Source: CAD feature listing. Evaluate the final solid. Frame: model axes, mm. Face numbers are marked on the shaded views. A direction names the side the tool comes from. Give positions to 0.01 mm unless a question says otherwise; leave off trailing zeros. Write each loop counter-clockwise with the first axis right and the second up, starting at its lowest first coordinate (ties: lowest second). Pieces come first, ordered by that corner, then holes. Notation, with made-up numbers: M 36.5,-2 L 74.5,-2 A26 cw 74.5,21 Z; hole C 72.5,67.5 d1. An arc over 180 degrees is marked long. Return JSON: item names as keys, results as strings.
```python
from build123d import *

# Parameters (mm, degrees)
F1_DEPTH = 30
F2_W     = 20
F2_H     = 20
F3_DEPTH = 20
F4_R     = 2
F5_W     = 6
F5_H     = 6
F6_DEPTH = 10
F7_R     = 2.9972
F8_R     = 1.9939
F9_DEPTH = 6


with BuildPart() as f1:
    # F0 (on Top) → F1 (new body)
    with BuildSketch(Plane.XY):
        Polygon((-21.213203, 21.213203), (0, 0), (21.213203, 21.213203), (0, 42.426407), align=None)
    extrude(amount=F1_DEPTH)

    # F2 (on face) → F3 (cut)
    with BuildSketch(Plane(origin=(0, 0, 0), x_dir=(0.707107, -0.707107, 0), z_dir=(-0.707107, -0.707107, 0))):
        with Locations((-15, 15)):
            Rectangle(F2_W, F2_H)
    extrude(amount=-F3_DEPTH, mode=Mode.SUBTRACT)

    # F4
    f4_edges = [f1.edges().sort_by_distance(p)[0] for p in [
        (0, 42.426407, 15),
        (-21.213203, 21.213203, 15),
        (-10.606602, 31.819805, 0),
        (-10.606602, 31.819805, 30),
        (-10.606602, 10.606602, 30),
        (10.606602, 10.606602, 30),
        (10.606602, 31.819805, 30),
        (0, 0, 15),
        (21.213203, 21.213203, 15),
        (10.606602, 10.606602, 0),
        (10.606602, 31.819805, 0),
        (-10.606602, 10.606602, 0),
    ]]
    fillet(f4_edges, radius=F4_R)

    # F5 (on face) → F6 (join)
    with BuildSketch(Plane(origin=(21.213203, 21.213203, 0), x_dir=(-0.707107, 0.707107, 0), z_dir=(0.707107, 0.707107, 0))):
        with Locations((15, 15)):
            Rectangle(F5_W, F5_H)
    extrude(amount=F6_DEPTH)

    # F7
    f7_edges = [f1.edges().sort_by_distance(p)[0] for p in [
        (19.79899, 36.769553, 15),
        (15.556349, 41.012193, 15),
    ]]
    fillet(f7_edges, radius=F7_R)

    # F8 (on face) → F9 (cut)
    with BuildSketch(Plane(origin=(0, 0, 12), x_dir=(1, 0, 0), z_dir=(0, 0, -1))):
        with Locations((15.556349, -36.773512)):
            Circle(F8_R)
    extrude(amount=-F9_DEPTH, mode=Mode.SUBTRACT)


solid = f1.part
```
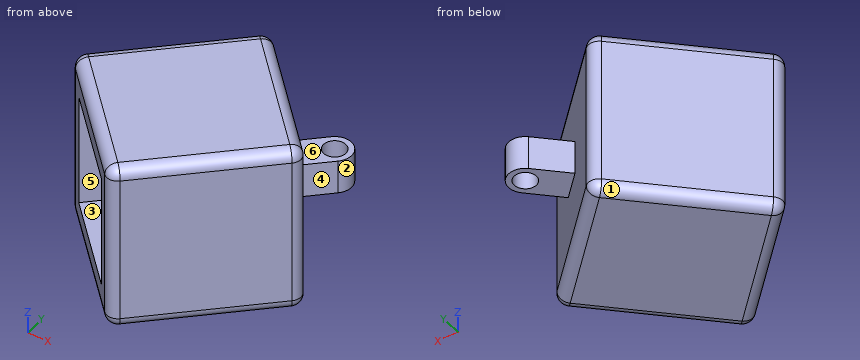
1) Contact query for flat-ended pins moving along their axis: pin 1 Ø6.5 at (x, y) = (15.56, 36.77) entering from -Z; pin 2 Ø6 at (x, z) = (10, 18.5) entering from +Y; pin 3 Ø2 at (x, z) = (-9.5, 25.5) entering from -Y; pin 4 Ø3 at (x, z) = (-1.5, 5.5) entering from -Y. Output: stop coordinate, or through.
Numbers:
{"pin 1": "stops at z = 12", "pin 2": "stops at y = 38.41", "pin 3": "stops at y = 8.5", "pin 4": "stops at y = 0.83"}
2) Set-up query: the marked faces 4, 5 and 6. Return all of +Z, -Z, +X, -X, +Y, -Y with unobstructed straight access to the full face (end or side cutting, diameter ignored); none if empty.
Numbers:
{"face 4": "+Z, -Z, +X", "face 5": "-Y", "face 6": "+Z, +X, +Y"}
3) Draft query along Z for the marked faces 1, 2 and 3. Return one class per face: released by +Z, released by -Z, zero draft, split by the parting line, or undercut.
Numbers:
{"face 1": "released by -Z", "face 2": "zero draft", "face 3": "undercut"}
4) Cut plane A-A, the plane z = 26.5. Return the cut outline in (x, y).
Numbers:
{"outline": "M -19.8,19.8 L -1.41,1.41 A2 ccw 1.41,1.41 L 19.8,19.8 A2 ccw 19.8,22.63 L 1.41,41.01 A2 ccw -1.41,41.01 L -19.8,22.63 A2 ccw Z"}
5) Line query: line 1 (Z direction, x = -1.5, y = 10.5); line 2 (Z direction, x = 12, y = 34); line 3 (Y direction, x = 7.5, z = 12). Output: solid intervals per line, ascending. Write a range as [from, to].
Numbers:
{"line 1": "z = [0, 5], [25, 30]", "line 2": "z = [12, 18]", "line 3": "y = [7.5, 14.57], [20.78, 34.93]"}
6) Cut plane B-B, the plane x = 17. Give the number of separate pieces and of enclosed holes in the cut face, then the cut area to 3 significant figures.
Numbers:
{"separate pieces": "3", "enclosed holes": "0", "area": "264 mm²"}
7) Cut plane C-C, the plane z = 11. Return the cut outline in (x, y).
Numbers:
{"outline": "M -19.8,19.8 L -17.68,17.68 L -3.54,31.82 L 10.61,17.68 L -3.54,3.54 L -1.41,1.41 A2 ccw 1.41,1.41 L 19.8,19.8 A2 ccw 19.8,22.63 L 1.41,41.01 A2 ccw -1.41,41.01 L -19.8,22.63 A2 ccw Z"}
